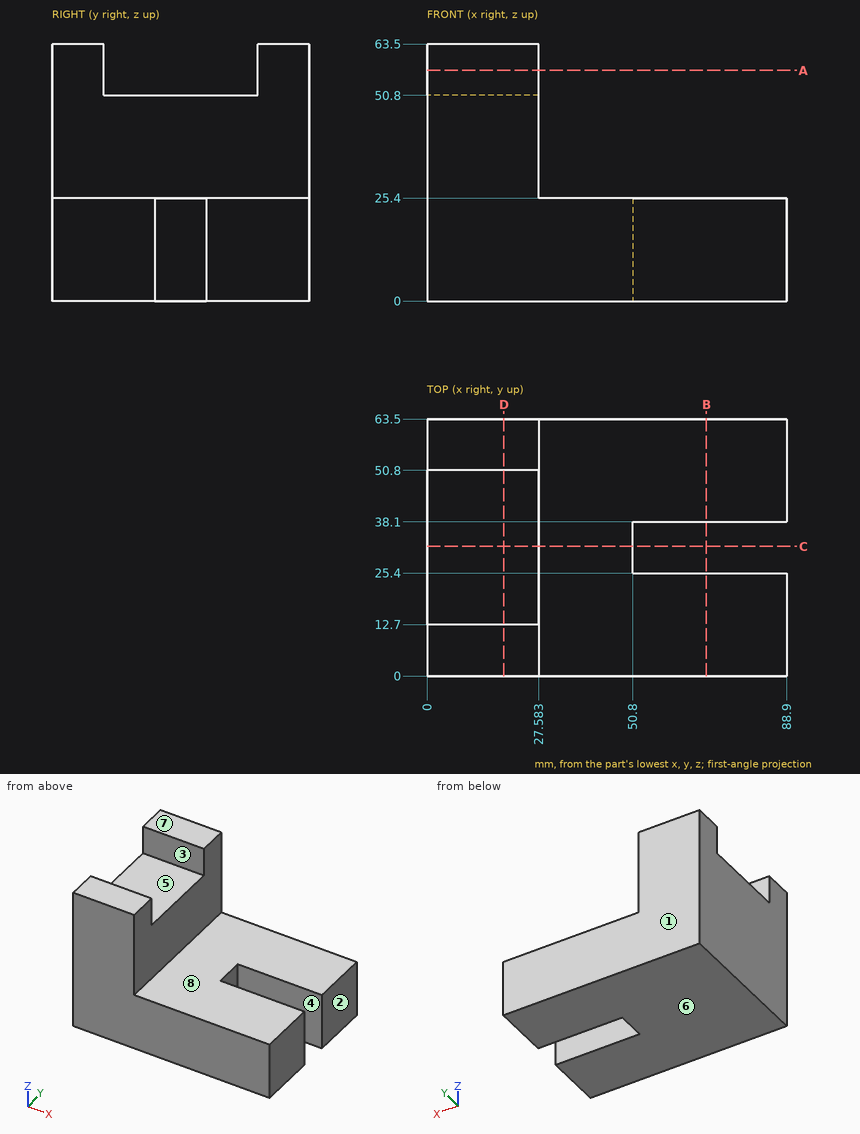
Study the drawing (mm; zero at the part's minimum x, y, z) and answer. A direction names the side the tool comes from. Coordinates: 2 decimals unless noted, no trailing zeros. Loops run counter-clockwise (first coordinate to the right, second up) from the corner with the lowest first, then second, coordinate; pieces in that order, holes last. Notation, with made-up numbers: (73, 33.25) -> (77, 33.25) arc R13 ccw to (77, 48.25) -> close; hole circle Ø3 at (87, 46.25). An arc over 180 degrees is marked (long way). Answer as CSV lines item,"result".
1) The part is cut by section A-A (z = 57). Give the vertices of the cut face in (x, y), and give its area (3 significant figures).
A:
outline,"(0, 0) -> (27.58, 0) -> (27.58, 12.7) -> (0, 12.7) -> close; (0, 50.8) -> (27.58, 50.8) -> (27.58, 63.5) -> (0, 63.5) -> close"
area,"701 mm²"
2) The part is cut by section C-C (y = 32). Give the vertices of the cut face in (x, z).
A:
outline,"(0, 0) -> (50.8, 0) -> (50.8, 25.4) -> (27.58, 25.4) -> (27.58, 50.8) -> (0, 50.8) -> close"
3) For the marked faces 4, 5, 6, 7 and 8, determine the directions among +Z, -Z, +X, -X, +Y, -Y from which every point of the face is accessible in a straight line to the end or side of a thin tool.
A:
face 4,"+Z, -Z, +X"
face 5,"+Z, +X, -X"
face 6,"-Z, +X, -X, +Y, -Y"
face 7,"+Z, +X, -X, +Y, -Y"
face 8,"+Z, +X, +Y, -Y"
4) Flat-ended cylindrical pins translate along their axes: pin 1 (10 mm diameter, centred on x = 56.5, z = 8.5, fed in from -Y); pin 2 (2 mm diameter, centred on y = 10.5, z = 41, fed in from +X); pin 3 (22 mm diameter, centred on x = 10.5, y = 34.5, fed in from +Z). Find the tip coordinate at first contact, or state that the pin passes through.
A:
pin 1,"stops at y = 0"
pin 2,"stops at x = 27.58"
pin 3,"stops at z = 50.8"
5) For a pull along Y with two mould halves and no side action, classify the marked faces 1, 2 and 3 as released by +Y, released by -Y, zero draft, split by the parting line, or undercut.
A:
face 1,"released by +Y"
face 2,"zero draft"
face 3,"undercut"
6) Straight lines are drawn through the part: probe 1 along X at (y, z) = (47, 30); probe 2 along Z at (x, y) = (61.5, 24); probe 3 along Y at (x, z) = (69, 5). For each, find the intervals that lie inside material, in ascending order.
A:
probe 1,"x = 0 to 27.58"
probe 2,"z = 0 to 25.4"
probe 3,"y = 0 to 25.4, 38.1 to 63.5"
7) The part is cut by section B-B (x = 69). Give the vertices of the cut face in (y, z).
A:
outline,"(0, 0) -> (25.4, 0) -> (25.4, 25.4) -> (0, 25.4) -> close; (38.1, 0) -> (63.5, 0) -> (63.5, 25.4) -> (38.1, 25.4) -> close"
8) The part is cut by section D-D (x = 19). Give the vertices of the cut face in (y, z), and give its area (3 significant figures).
A:
outline,"(0, 0) -> (63.5, 0) -> (63.5, 63.5) -> (50.8, 63.5) -> (50.8, 50.8) -> (12.7, 50.8) -> (12.7, 63.5) -> (0, 63.5) -> close"
area,"3,550 mm²"
